Geometry: final body of the model. Coordinates: model frame, mm. A direction names the side the tool comes from. Give positions to 0.01 mm unless a question says otherwise; leave off trailing zeros. Order: outer loops, then holes, each group sorted by start corner. A loop starts at its lowest first (then second) coordinate and runs counter-clockwise, first axis right, second up. Notation, with made-up numbers: (-14.75, 49) - (11.25, 49) arc R34 cw to (11.25, 81) - close; hole circle Ø8 at (78, 37). An arc over 180 degrees is marked (long way). Put each result on its own line as item: value. Start each with the question number.
1. Mould query, pull axis Y, two halves, no side actions, for faces 3 (the cylindrical face through (-2.75, -12.4, -0.02)), 4 (the flat face through (3, -3, -3.175)), 5 (the cylindrical face through (5.595, -3.569, -0.044)). Classes: pulls with the +Y half, pulls with the -Y half, needs draft (parallel to the pull), parting line crosses it, or undercut.
2. Set-up query: faces 1 (the cylindrical face through (-0.245, -7.571, 1.103)), 2 (the flat face through (3, -3, 3.175)). Return all of +Z, -Z, +X, -X, +Y, -Y with unobstructed straight access to the full face (end or side cutting, diameter ignored); none if empty.
3. First-contact query: P1, Ø1, axis at y = -5.5, z = 0.5, coming from the +X side; P2, Ø1.6, axis at x = 6.89, y = -3.98, coming from the +Z side; P3, Ø3, axis at x = -2, z = 2.5, coming from the +Y side. Flat tips, straight axial feed; report the tip coordinate or a pass-through.
4. Section A-A on y = 0. Return the cut outline in (x, z) (3 decimals).
5. Section B-B on x = 0. Return the cut outline in (y, z) (3 decimals).
6. Ray query, line 1 along Y through (x, z) = (0, -1) (3 decimals); line 2 along X through (y, z) = (-3.75, 0.5); line 3 along X through (y, z) = (-3.5, 0). Return the intervals inside material, ascending. Write a range as from..to.
7. Section C-C on z = 0. Return the cut outline in (x, y) (3 decimals), plus the area to 3 significant figures.
from build123d import *
from OCP.BRepFilletAPI import BRepFilletAPI_MakeChamfer

# Parameters (mm, degrees)
SKETCH2_R             = 12.7
SKETCH2_R_2           = 3.175
BOSS_EXTRUDE1_DEPTH   = 3.175
CHAMFER1_SIZE         = 0.254
CHAMFER1_SIZE2        = 0.132224031
F_6_32_TAPPED_HOLE1_D = 2.7051


# Read off the part's stored shape, not the designer's step: #4-40 Tapped Hole2
with BuildPart() as part:
    # Sketch2 → Boss-Extrude1 (new, symmetric)
    with BuildSketch(Plane.XY):
        Circle(SKETCH2_R)
        Circle(SKETCH2_R_2, mode=Mode.SUBTRACT)
    extrude(amount=BOSS_EXTRUDE1_DEPTH, both=True)

    # Chamfer1: one chamfer whose edges measure the first distance from different faces: ONE call of the kernel's chamfer builder (chamfer() names one face for all edges)
    chamfer1_edges_1 = [part.edges().sort_by_distance(p)[0] for p in [
        (-12.7, 0, -3.175),
    ]]
    chamfer1_side_1 = [part.faces().sort_by_distance(p)[0] for p in [
        (-12.340789755, 0, -3.175),
    ]]
    chamfer1_edges_2 = [part.edges().sort_by_distance(p)[0] for p in [
        (-12.7, 0, 3.175),
    ]]
    chamfer1_side_2 = [part.faces().sort_by_distance(p)[0] for p in [
        (-12.7, 0, 0),
    ]]
    chamfer1 = BRepFilletAPI_MakeChamfer(part.part.solid().wrapped)
    for e in chamfer1_edges_1:
        chamfer1.Add(CHAMFER1_SIZE, CHAMFER1_SIZE2, e.wrapped, chamfer1_side_1[0].wrapped)  # the first distance lies on this face
    for e in chamfer1_edges_2:
        chamfer1.Add(CHAMFER1_SIZE, CHAMFER1_SIZE2, e.wrapped, chamfer1_side_2[0].wrapped)  # the first distance lies on this face
    add(Compound.cast(chamfer1.Shape()), mode=Mode.REPLACE)

    # #6-32 Tapped Hole1 (through all)
    with Locations(Plane.XY.offset(3.175)):
        with Locations((0, 7.9502), (6.885075165, -3.9751), (-6.885075165, -3.9751)):
            Hole(F_6_32_TAPPED_HOLE1_D / 2)

    # #4-40 Tapped Hole2 outline → #4-40 Tapped Hole2 (revolve, cut)
    with BuildSketch(Plane.XY):
        Polygon((0, -12.700018831), (1.473216369, -12.700018831), (1.1303, -12.305538673), (1.1303, -2.966966147), (0, -2.966966147), align=None)
    revolve(axis=Axis((0, 0, 0), (0, 1, 0)), mode=Mode.SUBTRACT)


solid = part.part
Resolved:
1. face 3: parting line crosses it
1. face 4: needs draft
1. face 5: undercut
2. face 1: -Y
2. face 2: +Z, +X, -X, +Y, -Y
3. P1: x = 11.67
3. P2: through
3. P3: y = 12.69
4. outline: (-12.7, -3.043) - (-12.446, -3.175) - (-3.175, -3.175) - (-3.175, 3.175) - (-12.568, 3.175) - (-12.7, 2.921) - close; (3.175, -3.175) - (12.446, -3.175) - (12.7, -3.043) - (12.7, 2.921) - (12.568, 3.175) - (3.175, 3.175) - close
5. outline: (-12.7, -3.043) - (-12.446, -3.175) - (-3.175, -3.175) - (-3.175, -1.13) - (-12.306, -1.13) - (-12.7, -1.473) - close; (-12.7, 1.473) - (-12.306, 1.13) - (-3.175, 1.13) - (-3.175, 3.175) - (-12.568, 3.175) - (-12.7, 2.921) - close; (3.175, -3.175) - (6.598, -3.175) - (6.598, 3.175) - (3.175, 3.175) - close; (9.303, -3.175) - (12.446, -3.175) - (12.7, -3.043) - (12.7, 2.921) - (12.568, 3.175) - (9.303, 3.175) - close
6. line 1: 3.175..6.598, 9.303..12.7
6. line 2: -12.13..-8.22, -5.55..-1.01, 1.01..5.55, 8.22..12.13
6. line 3: -12.21..-8.15, -5.62..-1.13, 1.13..5.62, 8.15..12.21
7. outline: (-1.405, -12.622) - (-1.13, -12.306) - (-1.13, -2.967) arc R3.175 cw (long way) to (1.13, -2.967) - (1.13, -12.306) - (1.405, -12.622) arc R12.7 ccw (long way) to start; hole circle Ø2.705 at (-6.885, -3.975); hole circle Ø2.705 at (0, 7.95); hole circle Ø2.705 at (6.885, -3.975)
7. area: 436 mm^2
